Could you check a few things on this model? Use its own coordinates, in mm. Face numbers are marked on the shaded views. Give positions to 0.01 mm unless a question says otherwise; leave off trailing zeros. Order: outer loops, then holes, each group sorted by start corner. A loop starts at its lowest first (then second) coordinate and runs counter-clockwise, first axis right, second up. Notation, with made-up numbers: (-26.5, -13.75) -> (-3.5, -13.75) arc R25 cw to (-3.5, 19.25) -> close; hole circle Ø5 at (51.5, -15.75). An arc over 180 degrees is marked (long way). One line per item, written item: value.
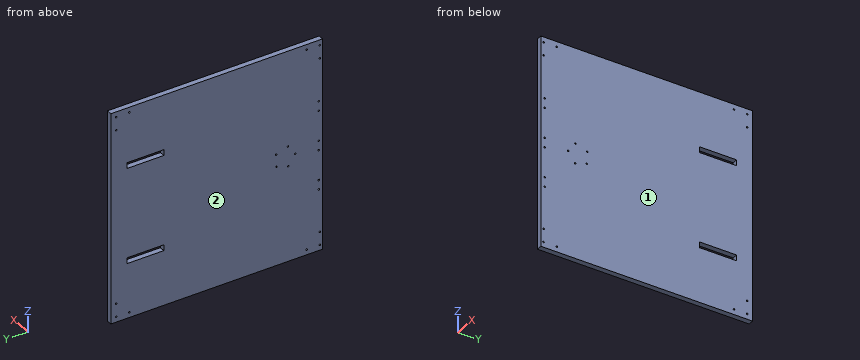
```python
from build123d import *

# Parameters (mm, degrees)
SKETCH_1_W          = 400
SKETCH_1_H          = 400
EXTRUDE_1_DEPTH     = 10
SKETCH_2_R          = 1.5
CUT_EXTRUDE_1_DEPTH = 10
SKETCH_3_R          = 1.5
CUT_EXTRUDE_2_DEPTH = 10
SKETCH_4_R          = 1.45
CUT_EXTRUDE_3_DEPTH = 10
SKETCH_5_W          = 11
SKETCH_5_H          = 70
CUT_EXTRUDE_5_DEPTH = 10


with BuildPart() as part:
    # 草图1 → 凸台-拉伸1 (new body)
    with BuildSketch(Plane(origin=(0, 0, 0), x_dir=(0, 0, -1), z_dir=(1, 0, 0))):
        Rectangle(SKETCH_1_W, SKETCH_1_H)
    extrude(amount=EXTRUDE_1_DEPTH)

    # 草图2 → 切除-拉伸1 (cut)
    with BuildSketch(Plane(origin=(10, 0, 0), x_dir=(0, 0, -1), z_dir=(1, 0, 0))):
        with Locations((190, 190)):
            Circle(SKETCH_2_R)
        with Locations((165, 190)):
            Circle(SKETCH_2_R)
        with Locations((190, 165)):
            Circle(SKETCH_2_R)
        with Locations((190, -195)):
            Circle(SKETCH_2_R)
        with Locations((165, -195)):
            Circle(SKETCH_2_R)
        with Locations((190, -170)):
            Circle(SKETCH_2_R)
    cut_extrude_1 = extrude(amount=-CUT_EXTRUDE_1_DEPTH, mode=Mode.SUBTRACT)

    # 草图3 → 切除-拉伸2 (cut)
    with BuildSketch(Plane(origin=(10, 0, 0), x_dir=(0, 0, -1), z_dir=(1, 0, 0))):
        with Locations((-84, -193)):
            Circle(SKETCH_3_R)
        with Locations((-66, -193)):
            Circle(SKETCH_3_R)
        with Locations((-9, -193)):
            Circle(SKETCH_3_R)
        with Locations((9, -193)):
            Circle(SKETCH_3_R)
        with Locations((66, -193)):
            Circle(SKETCH_3_R)
        with Locations((84, -193)):
            Circle(SKETCH_3_R)
    extrude(amount=-CUT_EXTRUDE_2_DEPTH, mode=Mode.SUBTRACT)

    # 镜向1: 切除-拉伸1 across plane
    add(cut_extrude_1.mirror(Plane.XY), mode=Mode.SUBTRACT)

    # 草图4 → 切除-拉伸3 (cut)
    with BuildSketch(Plane(origin=(10, 0, 0), x_dir=(0, 0, -1), z_dir=(1, 0, 0))):
        with Locations((-11.007896697, -112.622517601)):
            Circle(SKETCH_4_R)
        with Locations((12.238028253, -113.022211572)):
            Circle(SKETCH_4_R)
        with Locations((-18.571414113, -134.607193773)):
            Circle(SKETCH_4_R)
        with Locations((19.041282557, -135.253912204)):
            Circle(SKETCH_4_R)
        with Locations((0, -148.59416485)):
            Circle(SKETCH_4_R)
    extrude(amount=-CUT_EXTRUDE_3_DEPTH, mode=Mode.SUBTRACT)

    # 草图5 → 切除-拉伸5 (cut)
    with BuildSketch(Plane(origin=(0, 0, 0), x_dir=(0, 0, -1), z_dir=(1, 0, 0))):
        with Locations((-90.5, 135)):
            Rectangle(SKETCH_5_W, SKETCH_5_H)
        with Locations((90.5, 135)):
            Rectangle(SKETCH_5_W, SKETCH_5_H)
    extrude(amount=CUT_EXTRUDE_5_DEPTH, mode=Mode.SUBTRACT)


solid = part.part
```
1) We'd pull the mould along X, two halves only. Please class the marked faces 1 and 2: +X half, -X half, draft (parallel to the pull), parting line (faces both ways), or undercut.
Answer below:
face 1: +X half
face 2: -X half
2) Suppose I cut it at A-A, the plane y = 156. Write out the boundary of the cut face in (x, z), then the cut area to 3 significant figures.
Answer below:
outline: (0, -200) -> (10, -200) -> (10, -96) -> (0, -96) -> close; (0, -85) -> (10, -85) -> (10, 85) -> (0, 85) -> close; (0, 96) -> (10, 96) -> (10, 200) -> (0, 200) -> close
area: 3,780 mm2
3) For P1, Ø2.5, axis at y = -170, z = -190, coming from the -X side, with a flat end and sliding along its axis, tell me the tip position at first contact or that it passes through.
Answer below:
P1: passes through
4) If I drill on line 1 along Z through (x, y) = (8, 190); line 2 along Z through (x, y) = (2.5, 165); line 3 along Y through (x, z) = (2.5, 190), over which ranges is the centre line in solid material (lowest first)?
Answer below:
line 1: z = -200 to -191.5, -188.5 to -166.5, -163.5 to 163.5, 166.5 to 188.5, 191.5 to 200
line 2: z = -200 to -191.5, -188.5 to -96, -85 to 85, 96 to 188.5, 191.5 to 200
line 3: y = -200 to -196.5, -193.5 to -171.5, -168.5 to 163.5, 166.5 to 188.5, 191.5 to 200
